Verification items for the finished model (mm, model axes). A direction names the side the tool comes from. Round coordinates to 2 decimals unless told otherwise and drop trailing zeros. Order: outer loops, then holes, each group sorted by start corner. A loop starts at its lowest first (then second) coordinate and runs counter-clockwise, first axis right, second up. Notation, with made-up numbers: M 77,33.25 L 117,33.25 A10 cw 117,37.25 Z; hole C 24.25,88.5 d4. An arc over 180 degrees is marked long. Use one line per item in the form item = value. Start each with the question number.
Item 1: Cross-section at C-C on x = 9. Enter the section's corners in (y, z), then the cut area to 3 significant figures.
Item 2: Release check for a two-part mould opening along X. For faces 4 (the cylindrical face through (-13.986, 0.616, 7.395)), 5 (the flat face through (5, 6, 15)), 6 (the flat face through (3, 6, 11)) record: +X half, -X half, draft (parallel to the pull), parting line (faces both ways), or undercut.
Item 3: Go/stop test with flat-tipped pins: pin 1 Ø1 at (x, z) = (-11.5, 14.5) entering from -Y; pin 2 Ø3 at (y, z) = (2, 10) entering from -X; pin 3 Ø12 at (x, y) = (-15, 7.5) entering from -Z; pin 4 Ø0.6 at (y, z) = (1.5, 14) entering from -X. Record where each tip stops, or that it passes through.
Item 4: Cross-section at A-A on x = 0. Enter the section's corners in (y, z), then the cut area to 3 significant figures.
Item 5: Tool access check on faces 1 (the flat face through (-11, 0.857, 14)), 2 (the cylindrical face through (12.6, 1.96, 5.42)), 3 (the flat face through (12.721, 1, 14)). Record the directions out of +Z, -Z, +X, -X, +Y, -Y that give a thin tool (end or side, any length) a straight path to the whole face; none if there is none.
Item 6: Cross-section at B-B on y = 10.5. Enter the section's corners in (x, z), then the cut area to 3 significant figures.
Item 7: Thickness scan on probe 1 along X at (y, z) = (0, 12.5); probe 2 along Y at (x, z) = (0, 8.75); probe 3 along X at (y, z) = (0, 14.35). Record the ranges inside material, lowest first. Write a range as [from, to].
Item 8: Cross-section at D-D on z = 13.75. Count the separate pieces of the cut face and the enclosed holes in it, then the cut area to 3 significant figures.
from build123d import *

# Parameters (mm, degrees)
IZIM7_R                     = 14
Y_KSEKLIK_EKSTR_ZYON3_DEPTH = 15
IZIM8_R                     = 12.75
KES_EKSTR_ZYON2_DEPTH       = 13
IZIM10_RX                   = 20.721224891
IZIM10_RY                   = 8.451844087
Y_KSEKLIK_EKSTR_ZYON5_DEPTH = 2
IZIM11_R                    = 1.5
KES_EKSTR_ZYON4_DEPTH       = 12
IZIM12_R                    = 1.39637185
KES_EKSTR_ZYON5_DEPTH       = 12
IZIM13_R                    = 1.39637185
KES_EKSTR_ZYON9_DEPTH       = 10
IZIM17_R                    = 6.48453934
KES_EKSTR_ZYON10_DEPTH      = 10
IZIM18_R                    = 12.75
Y_KSEKLIK_EKSTR_ZYON6_DEPTH = 2
IZIM19_R                    = 6.48453934
KES_EKSTR_ZYON11_DEPTH      = 15
IZIM20_W                    = 4.233334515
IZIM20_H                    = 2.828390799
KES_EKSTR_ZYON12_DEPTH      = 15


with BuildPart() as part:
    # Çizim7 → Yükseklik-Ekstrüzyon3 (new body)
    with BuildSketch(Plane.XY):
        Circle(IZIM7_R)
    extrude(amount=Y_KSEKLIK_EKSTR_ZYON3_DEPTH)

    # Çizim8 → Kes-Ekstrüzyon2 (cut)
    with BuildSketch(Plane(origin=(0, 0, 0), x_dir=(-1, 0, 0), z_dir=(0, 0, -1))):
        Circle(IZIM8_R)
    extrude(amount=-KES_EKSTR_ZYON2_DEPTH, mode=Mode.SUBTRACT)

    # Çizim10 → Yükseklik-Ekstrüzyon5 (add)
    with BuildSketch(Plane.XY.offset(15)):
        with Locations(Location((0, 0), (0, 0, -177.201101486))):
            Ellipse(IZIM10_RX, IZIM10_RY)
    extrude(amount=-Y_KSEKLIK_EKSTR_ZYON5_DEPTH)

    # Çizim11 → Kes-Ekstrüzyon4 (cut)
    with BuildSketch(Plane(origin=(0, 0, 13), x_dir=(-1, 0, 0), z_dir=(0, 0, -1))):
        with Locations((-17.700084822, 0.922540909)):
            Circle(IZIM11_R)
        with Locations((17.700084822, -0.808134051)):
            Circle(IZIM11_R)
    extrude(amount=-KES_EKSTR_ZYON4_DEPTH, mode=Mode.SUBTRACT)

    # Çizim12 → Kes-Ekstrüzyon5 (cut)
    with BuildSketch(Plane(origin=(0, 0, 13), x_dir=(-1, 0, 0), z_dir=(0, 0, -1))):
        with Locations((-11.340835644, 0.538812648)):
            Circle(IZIM12_R)
        with Locations((11.231387984, -0.55728261)):
            Circle(IZIM12_R)
    extrude(amount=-KES_EKSTR_ZYON5_DEPTH, mode=Mode.SUBTRACT)

    # Çizim13 → Kes-Ekstrüzyon9 (cut)
    with BuildSketch(Plane(origin=(0, 0, 13), x_dir=(-1, 0, 0), z_dir=(0, 0, -1))):
        with BuildLine():
            Line((8.487842828, 0.857001804), (8.487842828, -1.971567024))
            Line((8.487842828, -1.971567024), (12.596643341, -1.971567024))
            ThreePointArc((12.596643341, -1.971567024), (12.671184838, -1.415476879), (12.721189334, -0.856645746))
            Line((12.721189334, -0.856645746), (12.721189334, 0.857001804))
            Line((12.721189334, 0.857001804), (8.487842828, 0.857001804))
        make_face()
        with Locations((11.231387984, -0.55728261)):
            Circle(IZIM13_R, mode=Mode.SUBTRACT)
        with BuildLine():
            Line((-12.721189334, 0.327914487), (-12.721189334, -0.856645746))
            Line((-12.721189334, -0.856645746), (-11.391335286, -0.856645746))
            ThreePointArc((-11.391335286, -0.856645746), (-12.269614978, -0.503887353), (-12.721189334, 0.327914487))
        make_face()
        with BuildLine():
            Line((-12.721189334, 1.971923081), (-12.721189334, 0.749710808))
            ThreePointArc((-12.721189334, 0.749710808), (-10.298135643, 1.467591981), (-11.290336002, -0.856645746))
            Line((-11.290336002, -0.856645746), (-8.487842828, -0.856645746))
            Line((-8.487842828, -0.856645746), (-8.487842828, 1.971923081))
            Line((-8.487842828, 1.971923081), (-12.721189334, 1.971923081))
        make_face()
    extrude(amount=-KES_EKSTR_ZYON9_DEPTH, mode=Mode.SUBTRACT)

    # Çizim17 → Kes-Ekstrüzyon10 (cut)
    with BuildSketch(Plane(origin=(0, 0, 13), x_dir=(-1, 0, 0), z_dir=(0, 0, -1))):
        Circle(IZIM17_R)
    extrude(amount=-KES_EKSTR_ZYON10_DEPTH, mode=Mode.SUBTRACT)

    # Çizim18 → Yükseklik-Ekstrüzyon6 (add)
    with BuildSketch(Plane(origin=(0, 0, 13), x_dir=(-1, 0, 0), z_dir=(0, 0, -1))):
        Circle(IZIM18_R)
    extrude(amount=Y_KSEKLIK_EKSTR_ZYON6_DEPTH)

    # Çizim19 → Kes-Ekstrüzyon11 (cut)
    with BuildSketch(Plane.XY.offset(13)):
        Circle(IZIM19_R)
    extrude(amount=-KES_EKSTR_ZYON11_DEPTH, mode=Mode.SUBTRACT)

    # Çizim20 → Kes-Ekstrüzyon12 (cut)
    with BuildSketch(Plane.XY.offset(15)):
        with Locations((-10.604510085, -0.557371624)):
            Rectangle(IZIM20_W, IZIM20_H)
    extrude(amount=-KES_EKSTR_ZYON12_DEPTH, mode=Mode.SUBTRACT)


solid = part.part
Output values:
q1.outline = M -10.72,0 L -9.03,0 L -9.03,11 L 9.03,11 L 9.03,0 L 10.72,0 L 10.72,15 L 1.97,15 L 1.97,13 L -0.86,13 L -0.86,15 L -10.72,15 Z
q1.area = 117 mm2
q2.face_4 = parting line
q2.face_5 = draft
q2.face_6 = undercut
q3.pin_1 = -8.66
q3.pin_2 = -13.99
q3.pin_3 = 0
q3.pin_4 = -20.1
q4.outline = M -14,0 L -12.75,0 L -12.75,11 L -6.48,11 L -6.48,15 L -14,15 Z; M 6.48,11 L 12.75,11 L 12.75,0 L 14,0 L 14,15 L 6.48,15 Z
q4.area = 87.6 mm2
q5.face_1 = +Z, -Z
q5.face_2 = -Z
q5.face_3 = +Z
q6.outline = M -9.26,0 L -7.23,0 L -7.23,11 L 7.23,11 L 7.23,0 L 9.26,0 L 9.26,15 L -9.26,15 Z
q6.area = 119 mm2
q7.probe_1 = [-14, -12.72], [-8.49, -6.48], [6.48, 14]
q7.probe_2 = [-14, -12.75], [12.75, 14]
q7.probe_3 = [-20.6, -18.96], [-16.44, -12.72], [-8.49, -6.48], [6.48, 8.49], [12.72, 16.52], [18.88, 20.6]
q8.separate_pieces = 1
q8.enclosed_holes = 5
q8.area = 575 mm2
